The listing builds one solid part. Answer for the finished solid, in the listing's coordinates (mm). A direction names the side the tool comes from. Coordinates: 2 decimals unless noted, no trailing zeros. Order: outer loops, then holes, each group sorted by start corner. A loop starts at its lowest first (then second) coordinate and runs counter-clockwise, first axis right, second up. Notation, with made-up numbers: (-19.75, 51) -> (32.25, 51) arc R7 ccw to (32.25, 60) -> close; hole circle Ø9 at (-26, 72.25). An arc over 180 degrees is marked (long way). Write item = value, one per line.
from build123d import *

# Parameters (mm, degrees)
SKETCH1_W           = 94
SKETCH1_H           = 74
BOSS_EXTRUDE1_DEPTH = 8
SKETCH3_W           = 8
SKETCH3_H           = 74
BOSS_EXTRUDE2_DEPTH = 89
SKETCH4_W           = 8
SKETCH4_H           = 74
BOSS_EXTRUDE3_DEPTH = 89
SKETCH7_W           = 97
SKETCH7_H           = 12
BOSS_EXTRUDE6_DEPTH = 41.8
SKETCH13_W          = 26.8
SKETCH13_H          = 82
CUT_EXTRUDE3_DEPTH  = 15
SKETCH19_R          = 1.5
CUT_EXTRUDE4_DEPTH  = 100
FILLET1_R           = 10
FILLET2_R           = 10
FILLET3_R           = 10
FILLET4_R           = 10
FILLET5_R           = 10
FILLET6_R           = 10
FILLET7_R           = 10
FILLET8_R           = 10


with BuildPart() as part:
    # Sketch1 → Boss-Extrude1 (new body)
    with BuildSketch(Plane.XY):
        Rectangle(SKETCH1_W, SKETCH1_H)
    extrude(amount=BOSS_EXTRUDE1_DEPTH)

    # Sketch3 → Boss-Extrude2 (add)
    with BuildSketch(Plane(origin=(0, 0, 0), x_dir=(-1, 0, 0), z_dir=(0, 0, -1))):
        with Locations((43, 0)):
            Rectangle(SKETCH3_W, SKETCH3_H)
    extrude(amount=BOSS_EXTRUDE2_DEPTH)

    # Sketch4 → Boss-Extrude3 (add)
    with BuildSketch(Plane(origin=(0, 0, 0), x_dir=(-1, 0, 0), z_dir=(0, 0, -1))):
        with Locations((-43, 0)):
            Rectangle(SKETCH4_W, SKETCH4_H)
    extrude(amount=BOSS_EXTRUDE3_DEPTH)

    # Sketch7 → Boss-Extrude6 (add)
    with BuildSketch(Plane(origin=(47, 0, 0), x_dir=(0, 0, -1), z_dir=(1, 0, 0))):
        with Locations((40.5, 31)):
            Rectangle(SKETCH7_W, SKETCH7_H)
    extrude(amount=BOSS_EXTRUDE6_DEPTH)

    # Sketch13 → Cut-Extrude3 (cut)
    with BuildSketch(Plane.XZ.offset(-25)):
        with Locations((67.9, -40.5)):
            Rectangle(SKETCH13_W, SKETCH13_H)
    extrude(amount=-CUT_EXTRUDE3_DEPTH, mode=Mode.SUBTRACT)

    # Sketch19 → Cut-Extrude4 (cut)
    with BuildSketch(Plane(origin=(47, 0, 0), x_dir=(0, 0, -1), z_dir=(1, 0, 0))):
        with Locations(Location((54, 21, 0), (0, 0, 90))):
            Circle(SKETCH19_R)
        with Locations(Location((29.5, -6, 0), (0, 0, 90))):
            Circle(SKETCH19_R)
        with Locations(Location((78.5, -6, 0), (0, 0, 90))):
            Circle(SKETCH19_R)
        with Locations(Location((54, -33, 0), (0, 0, 90))):
            Circle(SKETCH19_R)
        with Locations(Location((54, -6, 0), (0, 0, 90))):
            Circle(SKETCH19_R)
    extrude(amount=-CUT_EXTRUDE4_DEPTH, mode=Mode.SUBTRACT)

    # Fillet1
    fillet1_edges = [part.edges().sort_by_distance(p)[0] for p in [
        (-43, 37, -89),
        (47, -6, 8),
    ]]
    fillet(fillet1_edges, radius=FILLET1_R)

    # Fillet2
    fillet2_edges = [part.edges().sort_by_distance(p)[0] for p in [
        (-43, -37, -89),
    ]]
    fillet(fillet2_edges, radius=FILLET2_R)

    # Fillet3
    fillet3_edges = [part.edges().sort_by_distance(p)[0] for p in [
        (43, -37, -89),
    ]]
    fillet(fillet3_edges, radius=FILLET3_R)

    # Fillet4
    fillet4_edges = [part.edges().sort_by_distance(p)[0] for p in [
        (-47, 0, 8),
    ]]
    fillet(fillet4_edges, radius=FILLET4_R)

    # Fillet5
    fillet5_edges = [part.edges().sort_by_distance(p)[0] for p in [
        (88.8, 31, 8),
    ]]
    fillet(fillet5_edges, radius=FILLET5_R)

    # Fillet6
    fillet6_edges = [part.edges().sort_by_distance(p)[0] for p in [
        (88.8, 31, -89),
    ]]
    fillet(fillet6_edges, radius=FILLET6_R)

    # Fillet7
    fillet7_edges = [part.edges().sort_by_distance(p)[0] for p in [
        (-39, 0, 0),
    ]]
    fillet(fillet7_edges, radius=FILLET7_R)

    # Fillet8
    fillet8_edges = [part.edges().sort_by_distance(p)[0] for p in [
        (39, 0, 0),
    ]]
    fillet(fillet8_edges, radius=FILLET8_R)


solid = part.part
Q1. Section A-A, the plane z = -23 is taken. Give the vertices of the cut face in (x, y).
The answers:
outline = (-47, -37) -> (-39, -37) -> (-39, 37) -> (-47, 37) -> close; (39, -37) -> (47, -37) -> (47, 25) -> (54.5, 25) -> (54.5, 37) -> (39, 37) -> close; (81.3, 25) -> (88.8, 25) -> (88.8, 37) -> (81.3, 37) -> close
Q2. Section B-B, the plane x = 65 is taken. Give the vertices of the cut face in (y, z).
The answers:
outline = (25, -89) -> (37, -89) -> (37, -81.5) -> (25, -81.5) -> close; (25, 0.5) -> (37, 0.5) -> (37, 8) -> (25, 8) -> close
Q3. Each of these flat-tipped pins is pushed along its axis until it touches: pin 1 Ø1.5 at (y, z) = (11.5, -69.5) entering from +X; pin 2 Ø1.8 at (y, z) = (21, -54) entering from +X; pin 3 Ø5 at (x, z) = (56.5, -70.5) entering from -Y; pin 4 Ø8 at (x, y) = (5, -21) entering from -Z. Where does it stop, or does it pass through?
The answers:
pin_1 = 47
pin_2 = through
pin_3 = 25
pin_4 = 0
Q4. Section D-D, the plane y = 21 is taken. Give the vertices of the cut face in (x, z), plus the area to 3 significant figures.
The answers:
outline = (-47, -89) -> (-39, -89) -> (-39, -55.5) -> (-47, -55.5) -> close; (-47, -52.5) -> (-39, -52.5) -> (-39, -10) arc R10 cw to (-29, 0) -> (29, 0) arc R10 cw to (39, -10) -> (39, -52.5) -> (47, -52.5) -> (47, -2) arc R10 ccw to (37, 8) -> (-37, 8) arc R10 ccw to (-47, -2) -> close; (39, -89) -> (47, -89) -> (47, -55.5) -> (39, -55.5) -> close
area = 2,130 mm2
Q5. The mould has two halves that part along X. Classify faces 1 (the face through (0, 1, 0)), 2 (the face through (41, 37, -29)), 3 (the face through (85.79, 31.08, 5.15)): released by +X, released by -X, zero draft, split by the parting line, or undercut.
The answers:
face_1 = undercut
face_2 = zero draft
face_3 = released by +X
Q6. Section C-C, the plane y = -33 is taken. Give the vertices of the cut face in (x, z).
The answers:
outline = (-47, -87) -> (-39, -87) -> (-39, -55.5) -> (-47, -55.5) -> close; (-47, -52.5) -> (-39, -52.5) -> (-39, -10) arc R10 cw to (-29, 0) -> (29, 0) arc R10 cw to (39, -10) -> (39, -52.5) -> (47, -52.5) -> (47, -2) arc R10 ccw to (37, 8) -> (-37, 8) arc R10 ccw to (-47, -2) -> close; (39, -87) -> (47, -87) -> (47, -55.5) -> (39, -55.5) -> close
Q7. Find the intervals of material crossed by line 1 along X through (y, z) = (26, -67.5); line 2 along Y through (x, z) = (-40.5, -78.5); line 3 along Z through (x, y) = (-41.25, -6), in increasing order.
The answers:
line_1 = -47 to -39, 39 to 54.5, 81.3 to 88.8
line_2 = -37 to -7.5, -4.5 to 37
line_3 = -89 to -80, -77 to -55.5, -52.5 to -31, -28 to 7.05
Q8. A tool of negligible diameter and unlimited length cuts with its end or side. For faces 4 (the face through (-43, -6, -28)), 5 (the face through (-35.99, 0.52, -2.85)), 6 (the face through (68, 31, -81.5)), from which of +Z, -Z, +X, -X, +Y, -Y can it reach the whole face along a straight path? Write none if from no direction.
The answers:
face_4 = +X, -X
face_5 = -Z, +Y, -Y
face_6 = +Y, -Y
